Geometry: final body of the model. Coordinates: model frame, mm. A direction names the side the tool comes from. Give positions to 0.01 mm unless a question says otherwise; leave off trailing zeros. Order: outer loops, then holes, each group sorted by start corner. A loop starts at its lowest first (then second) coordinate and runs counter-clockwise, first axis right, second up. Notation, with made-up numbers: (11.5, -30.5) -> (51.5, -30.5) arc R10 ccw to (51.5, -20.5) -> close; hole circle Ø10 at (-38.75, -4.75). An arc over 180 degrees is marked (long way). One line per question, with ' | ' between items.
from build123d import *

# Parameters (mm, degrees)
F0_R     = 53.975
F1_DEPTH = 4.7625
F2_D     = 3.175
F2_DEPTH = 9.525


with BuildPart() as f1:
    # F0 (on Top) → F1 (new body)
    with BuildSketch(Plane.XY):
        with BuildLine():
            ThreePointArc((0, -84.829008), (46.583097, -119.764619), (102.051281, -102.051281))
            ThreePointArc((102.051281, -102.051281), (119.764619, -46.583097), (84.829008, 0))
            ThreePointArc((84.829008, 0), (119.764619, 46.583097), (102.051281, 102.051281))
            ThreePointArc((102.051281, 102.051281), (46.583097, 119.764619), (0, 84.829008))
            ThreePointArc((0, 84.829008), (-46.583097, 119.764619), (-102.051281, 102.051281))
            ThreePointArc((-102.051281, 102.051281), (-119.764619, 46.583097), (-84.829008, 0))
            ThreePointArc((-84.829008, 0), (-119.764619, -46.583097), (-102.051281, -102.051281))
            ThreePointArc((-102.051281, -102.051281), (-46.583097, -119.764619), (0, -84.829008))
        make_face()
        with BuildLine():
            ThreePointArc((-3.175, -57.15), (-36.494662, -107.016398), (-95.316089, -95.316089))
            ThreePointArc((-95.316089, -95.316089), (-77.805338, -7.283602), (-3.175, -57.15))
        make_face(mode=Mode.SUBTRACT)
        with BuildLine():
            ThreePointArc((95.316089, -95.316089), (7.283602, -36.494662), (111.125, -57.15))
            ThreePointArc((111.125, -57.15), (107.016398, -77.805338), (95.316089, -95.316089))
        make_face(mode=Mode.SUBTRACT)
        Polygon((-29.470992, 0), (0, 29.470992), (29.470992, 0), (0, -29.470992), align=None, mode=Mode.SUBTRACT)
        with Locations((-57.15, 57.15)):
            Circle(F0_R, mode=Mode.SUBTRACT)
        with Locations((57.15, 57.15)):
            Circle(F0_R, mode=Mode.SUBTRACT)
    extrude(amount=F1_DEPTH)

    # F2
    with Locations(Plane(origin=(0, 0, 0), x_dir=(1, 0, 0), z_dir=(0, 0, -1))):
        with Locations((-98.683685, -98.683685), (-78.479008, 0), (-98.683685, 98.683685), (0, 78.479008), (98.683685, 98.683685), (78.479008, 0), (98.683685, -98.683685), (0, -78.479008)):
            Hole(F2_D / 2, depth=F2_DEPTH)


solid = f1.part
1) Section D-D on x = -11. Return loops of the section in (y, z), plus the area to 3 significant figures.
Check result:
outline: (-100.77, 0) -> (-85.14, 0) -> (-85.14, 4.76) -> (-100.77, 4.76) -> close; (-29.16, 0) -> (-18.47, 0) -> (-18.47, 4.76) -> (-29.16, 4.76) -> close; (18.47, 0) -> (29.16, 0) -> (29.16, 4.76) -> (18.47, 4.76) -> close; (85.14, 0) -> (100.77, 0) -> (100.77, 4.76) -> (85.14, 4.76) -> close | area: 251 mm^2
2) Material intervals for probe 1 along Y at (x, z) = (-57.15, 3.55) (3 decimals); probe 2 along Y at (x, z) = (-28, 1.85); probe 3 along X at (y, z) = (33.5, 2.1), sorted ascending. Write a range as from..to.
Check result:
probe 1: y = -120.65..-111.125, -3.175..3.175, 111.125..120.65 | probe 2: y = -113.56..-102.58, -11.72..-1.47, 1.47..11.72, 102.58..113.56 | probe 3: x = -116.08..-105.67, -8.63..8.63, 105.67..116.08
3) Contact query for flat-ended pins moving along their axis: pin 1 Ø2 at (x, z) = (24, 3.5) entering from -Y; pin 2 Ø1 at (y, z) = (56, 2.5) entering from -X; pin 3 Ø1 at (y, z) = (34, 1.5) entering from +X. Output: stop coordinate, or through.
Check result:
pin 1: stops at y = -111.91 | pin 2: stops at x = -120.65 | pin 3: stops at x = 116.47
4) Pull-direction query (Y, two-part tool) for faces 1 (the flat face through (14.53, 14.94, 2.35)), 2 (the flat face through (17, -17, 0)); classes: +Y half, -Y half, draft (parallel to the pull), parting line (faces both ways), or undercut.
Check result:
face 1: undercut | face 2: draft
5) Section C-C on y = -20. Return loops of the section in (x, z).
Check result:
outline: (-108.65, 0) -> (-96.31, 0) -> (-96.31, 4.76) -> (-108.65, 4.76) -> close; (-17.99, 0) -> (-9.47, 0) -> (-9.47, 4.76) -> (-17.99, 4.76) -> close; (9.47, 0) -> (17.99, 0) -> (17.99, 4.76) -> (9.47, 4.76) -> close; (96.31, 0) -> (108.65, 0) -> (108.65, 4.76) -> (96.31, 4.76) -> close
6) Set-up query: faces 3 (the flat face through (17, -17, 4.762)), 4 (the flat face through (14.94, -14.53, 2.35)). Return all of +Z, -Z, +X, -X, +Y, -Y with unobstructed straight access to the full face (end or side cutting, diameter ignored); none if empty.
Check result:
face 3: +Z, +X, -X, +Y, -Y | face 4: +Z, -Z
7) Section A-A on x = 57.15. Count the separate pieces of the cut face and the enclosed holes in it, plus the area to 3 significant figures.
Check result:
separate pieces: 3 | enclosed holes: 0 | area: 121 mm^2
